```python
from build123d import *

# Parameters (mm, degrees)
BOSS_EXTRUDE1_DEPTH     = 40
CUT_EXTRUDE2_DEPTH      = 58
CUT_EXTRUDE2_DEPTH_BACK = 4
FILLET2_R               = 50
SKETCH4_R               = 8
CUT_EXTRUDE4_DEPTH      = 58
CUT_EXTRUDE4_DEPTH_BACK = 4
CUT_EXTRUDE5_DEPTH      = 113
CUT_EXTRUDE5_DEPTH_BACK = 4


with BuildPart() as part:
    # Sketch1 → Boss-Extrude1 (new body, symmetric)
    with BuildSketch(Plane.YZ):
        with BuildLine():
            Line((8, 0), (115, 0))
            Line((115, 0), (115, 3))
            Line((115, 3), (8, 3))
            ThreePointArc((8, 3), (4.464466094, 4.464466094), (3, 8))
            Line((3, 8), (3, 56.75))
            ThreePointArc((3, 56.75), (3.25, 57), (3.5, 56.75))
            Line((3.5, 56.75), (3.5, 40))
            Line((3.5, 40), (6.5, 40))
            Line((6.5, 40), (6.5, 56.75))
            ThreePointArc((6.5, 56.75), (3.25, 60), (0, 56.75))
            Line((0, 56.75), (0, 8))
            ThreePointArc((0, 8), (2.343145751, 2.343145751), (8, 0))
        make_face()
    extrude(amount=BOSS_EXTRUDE1_DEPTH, both=True)

    # Sketch2 → Cut-Extrude2 (cut, two sides)
    with BuildSketch(Plane.XY.offset(3)) as cut_extrude2_sk:
        with BuildLine():
            Line((-135.973206715, -127.551210724), (-40, 56.811604044))
            Line((-40, 56.811604044), (-14.192173331, 106.387977812))
            ThreePointArc((-14.192173331, 106.387977812), (0, 115), (14.192173331, 106.387977812))
            Line((14.192173331, 106.387977812), (40, 56.811604044))
            Line((40, 56.811604044), (135.973206715, -127.551210724))
            Line((135.973206715, -127.551210724), (135.973206715, 288.143407362))
            Line((135.973206715, 288.143407362), (-135.973206715, 288.143407362))
            Line((-135.973206715, 288.143407362), (-135.973206715, -127.551210724))
        make_face()
    extrude(amount=CUT_EXTRUDE2_DEPTH, mode=Mode.SUBTRACT)
    extrude(cut_extrude2_sk.sketch, amount=-CUT_EXTRUDE2_DEPTH_BACK, mode=Mode.SUBTRACT)

    # Fillet2
    fillet2_edges = [part.edges().sort_by_distance(p)[0] for p in [
        (-40, 56.811604044, 1.5),
        (40, 56.811604044, 1.5),
    ]]
    fillet(fillet2_edges, radius=FILLET2_R)

    # Sketch4 → Cut-Extrude4 (cut, two sides)
    with BuildSketch(Plane.XY.offset(3)) as cut_extrude4_sk:
        with Locations((0, 99)):
            Circle(SKETCH4_R)
        with BuildLine():
            Line((4, 99), (4, 77))
            ThreePointArc((4, 77), (0, 73), (-4, 77))
            Line((-4, 77), (-4, 99))
            ThreePointArc((-4, 99), (0, 103), (4, 99))
        make_face()
    extrude(amount=CUT_EXTRUDE4_DEPTH, mode=Mode.SUBTRACT)
    extrude(cut_extrude4_sk.sketch, amount=-CUT_EXTRUDE4_DEPTH_BACK, mode=Mode.SUBTRACT)

    # Sketch5 → Cut-Extrude5 (cut, two sides)
    with BuildSketch(Plane(origin=(0, 3, 0), x_dir=(-1, 0, 0), z_dir=(0, 1, 0))) as cut_extrude5_sk:
        with BuildLine():
            Line((-20, 14), (20, 14))
            ThreePointArc((20, 14), (23.535533906, 15.464466094), (25, 19))
            Line((25, 19), (25, 29))
            ThreePointArc((25, 29), (23.535533906, 32.535533906), (20, 34))
            Line((20, 34), (-20, 34))
            ThreePointArc((-20, 34), (-23.535533906, 32.535533906), (-25, 29))
            Line((-25, 29), (-25, 19))
            ThreePointArc((-25, 19), (-23.535533906, 15.464466094), (-20, 14))
        make_face()
    extrude(amount=CUT_EXTRUDE5_DEPTH, mode=Mode.SUBTRACT)
    extrude(cut_extrude5_sk.sketch, amount=-CUT_EXTRUDE5_DEPTH_BACK, mode=Mode.SUBTRACT)


solid = part.part
```
Input: part model. Units: mm. Frame: model coordinates. A direction names the side the tool comes from. Give positions to 0.01 mm unless a question says otherwise; leave off trailing zeros. Loops run counter-clockwise (first coordinate to the right, second up) from the corner with the lowest first, then second, coordinate; pieces in that order, holes last. Notation, with made-up numbers: (64, 23.5) -> (119, 23.5) arc R18 cw to (119, 53.5) -> close; hole circle Ø1 at (25, 74.5). An arc over 180 degrees is marked (long way). Use a Markdown table: item, result.
Q1. Access query for faces 1 (the cylindrical face through (24, 2, 16)), 2 (the flat face through (1, 3.5, 48)), 3 (the flat face through (1, 50, 3)). Directions: +Z, -Z, +X, -X, +Y, -Y. A direction counts if a zero-diameter tool reaches every point of the face in a straight line with its end or side. Return the directions, or none.
Entries:
| item | result |
|---|---|
| face 1 | +Y, -Y |
| face 2 | +X, -X |
| face 3 | +Z, +X, -X, +Y |
Q2. Section query A-A, the plane x = 10. Return the cut outline in (y, z).
Entries:
| item | result |
|---|---|
| outline | (0, 8) arc R8 ccw to (8, 0) -> (111.49, 0) -> (111.49, 3) -> (8, 3) arc R5 cw to (3, 8) -> (3, 14) -> (0, 14) -> close; (0, 34) -> (3, 34) -> (3, 56.75) arc R0.25 cw to (3.5, 56.75) -> (3.5, 40) -> (6.5, 40) -> (6.5, 56.75) arc R3.25 ccw to (0, 56.75) -> close |
Q3. Pull-direction query (Z, two-part tool) for faces 4 (the flat face through (-25, 2, 24)), 5 (the cylindrical face through (0, 73, 2)), 6 (the cylindrical face through (0.6, 3.3, 60)); classes: pulls with the +Z half, pulls with the -Z half, needs draft (parallel to the pull), parting line crosses it, or undercut.
Entries:
| item | result |
|---|---|
| face 4 | undercut |
| face 5 | needs draft |
| face 6 | pulls with the +Z half |
Q4. Section query D-D, the plane y = 99. Return the cut outline in (x, z).
Entries:
| item | result |
|---|---|
| outline | (-18.04, 0) -> (-8, 0) -> (-8, 3) -> (-18.04, 3) -> close; (8, 0) -> (18.04, 0) -> (18.04, 3) -> (8, 3) -> close |
Q5. Section query C-C, the plane x = 0. Return the cut outline in (y, z), plus the area to 3 significant figures.
Entries:
| item | result |
|---|---|
| outline | (0, 8) arc R8 ccw to (8, 0) -> (73, 0) -> (73, 3) -> (8, 3) arc R5 cw to (3, 8) -> (3, 14) -> (0, 14) -> close; (0, 34) -> (3, 34) -> (3, 56.75) arc R0.25 cw to (3.5, 56.75) -> (3.5, 40) -> (6.5, 40) -> (6.5, 56.75) arc R3.25 ccw to (0, 56.75) -> close; (107, 0) -> (115, 0) -> (115, 3) -> (107, 3) -> close |
| area | 403 mm² |
Q6. First-contact query: P1, Ø0.9, axis at y = 81.5, z = 1, coming from the +X side; P2, Ø4, axis at x = 27.5, z = 27, coming from the -Y side; P3, Ø2.5, axis at x = -8.5, y = 1, coming from the +Z side; P4, Ø3, axis at x = -4.5, z = 10.5, coming from the +Y side. Flat tips, straight axial feed; report the tip coordinate or a pass-through.
Entries:
| item | result |
|---|---|
| P1 | stops at x = 27.38 |
| P2 | stops at y = 0 |
| P3 | stops at z = 59.84 |
| P4 | stops at y = 3 |
Q7. Section query B-B, the plane z = 55. Return the cut outline in (x, y), plus the area to 3 significant figures.
Entries:
| item | result |
|---|---|
| outline | (-40, 0) -> (40, 0) -> (40, 3) -> (-40, 3) -> close; (-40, 3.5) -> (40, 3.5) -> (40, 6.5) -> (-40, 6.5) -> close |
| area | 480 mm² |
Q8. Ray query, probe 1 along Y at (x, z) = (32, 50.5); probe 2 along Y at (x, z) = (0, 1.4); probe 3 along Z at (x, y) = (-4.5, 86.5). Return the intervals inside material, ascending. Write a range as from..to.
Entries:
| item | result |
|---|---|
| probe 1 | y = 0..3, 3.5..6.5 |
| probe 2 | y = 3.48..73, 107..115 |
| probe 3 | z = 0..3 |
